Check sheet for the modelled part. Datum: model origin and axes. Units: mm. A direction names the side the tool comes from. Round coordinates to 2 decimals unless told otherwise and drop trailing zeros. Write each loop counter-clockwise with the first axis right and the second up, starting at its lowest first coordinate (ties: lowest second). Pieces come first, ordered by that corner, then holes. Notation, with made-up numbers: (37, 32) -> (73, 32) arc R23 ccw to (73, 64) -> close; hole circle Ø1 at (-28, 80.25). An arc over 180 degrees is marked (long way). One line per item, written item: value.
from build123d import *

# Parameters (mm, degrees)
BOSS_EXTRUDE1_DEPTH = 3.81
BOSS_EXTRUDE3_DEPTH = 21.59
BOSS_EXTRUDE4_DEPTH = 2.54
FILLET1_R           = 2.54
BOSS_EXTRUDE6_DEPTH = 2.54
SKETCH9_R           = 1.905
CUT_EXTRUDE1_DEPTH  = 2.54
CUT_EXTRUDE2_DEPTH  = 1.27
SKETCH11_W          = 22.86
SKETCH11_H          = 2.54
CUT_EXTRUDE3_DEPTH  = 1.27
SKETCH12_W          = 22.86
SKETCH12_H          = 2.54
CUT_EXTRUDE4_DEPTH  = 1.27


with BuildPart() as part:
    # Sketch1 → Boss-Extrude1 (new body)
    with BuildSketch(Plane.XY):
        with BuildLine():
            Line((0, 62.289610149), (0, 73.614735329))
            Line((0, 73.614735329), (-19.541270744, 73.614735329))
            ThreePointArc((-19.541270744, 73.614735329), (-21.690891162, 73.166710129), (-22.687990425, 71.210339105))
            Line((-22.687990425, 71.210339105), (-20.412160003, 5.212586245))
            ThreePointArc((-20.412160003, 5.212586245), (-19.78310781, 3.39559701), (-18.061159176, 2.539998129))
            Line((-18.061159176, 2.539998129), (0, 2.539998129))
            Line((0, 2.539998129), (0, 8.872308918))
            ThreePointArc((0, 8.872308918), (-12.75, 21.622308918), (0, 34.372308918))
            Line((0, 34.372308918), (0, 54.789610149))
            ThreePointArc((0, 54.789610149), (-3.75, 58.539610149), (0, 62.289610149))
        make_face()
        with BuildLine():
            Line((20.141804619, 73.614735329), (0, 73.614735329))
            Line((0, 73.614735329), (0, 62.289610149))
            ThreePointArc((0, 62.289610149), (2.651650429, 61.191260578), (3.75, 58.539610149))
            ThreePointArc((3.75, 58.539610149), (2.651650429, 55.887959719), (0, 54.789610149))
            Line((0, 54.789610149), (0, 34.372308918))
            ThreePointArc((0, 34.372308918), (9.01561146, 30.637920378), (12.75, 21.622308918))
            ThreePointArc((12.75, 21.622308918), (9.01561146, 12.606697458), (0, 8.872308918))
            Line((0, 8.872308918), (0, 2.539998129))
            Line((0, 2.539998129), (17.866078187, 2.539998129))
            ThreePointArc((17.866078187, 2.539998129), (19.630909441, 3.253260423), (20.404569365, 4.992462187))
            Line((20.404569365, 4.992462187), (22.680295797, 70.987199387))
            ThreePointArc((22.680295797, 70.987199387), (21.968542325, 72.839566583), (20.141804619, 73.614735329))
        make_face()
        with BuildLine():
            Line((0, 76.154735329), (-22.77090231, 76.154735329))
            ThreePointArc((-22.77090231, 76.154735329), (-24.597640016, 75.379566583), (-25.309393487, 73.527199387))
            Line((-25.309393487, 73.527199387), (-22.858491178, 2.452464058))
            ThreePointArc((-22.858491178, 2.452464058), (-22.084831254, 0.713262294), (-20.32, 0))
            Line((-20.32, 0), (0, 0))
            Line((0, 0), (0, 2.539998129))
            Line((0, 2.539998129), (-18.061159176, 2.539998129))
            ThreePointArc((-18.061159176, 2.539998129), (-19.78310781, 3.39559701), (-20.412160003, 5.212586245))
            Line((-20.412160003, 5.212586245), (-22.687990425, 71.210339105))
            ThreePointArc((-22.687990425, 71.210339105), (-21.690891162, 73.166710129), (-19.541270744, 73.614735329))
            Line((-19.541270744, 73.614735329), (0, 73.614735329))
            Line((0, 73.614735329), (0, 76.154735329))
        make_face()
        with BuildLine():
            Line((22.77090231, 76.154735329), (0, 76.154735329))
            Line((0, 76.154735329), (0, 73.614735329))
            Line((0, 73.614735329), (20.141804619, 73.614735329))
            ThreePointArc((20.141804619, 73.614735329), (21.968542325, 72.839566583), (22.680295797, 70.987199387))
            Line((22.680295797, 70.987199387), (20.404569365, 4.992462187))
            ThreePointArc((20.404569365, 4.992462187), (19.630909441, 3.253260423), (17.866078187, 2.539998129))
            Line((17.866078187, 2.539998129), (0, 2.539998129))
            Line((0, 2.539998129), (0, 0))
            Line((0, 0), (20.32, 0))
            ThreePointArc((20.32, 0), (22.084831254, 0.713262294), (22.858491178, 2.452464058))
            Line((22.858491178, 2.452464058), (25.309393487, 73.527199387))
            ThreePointArc((25.309393487, 73.527199387), (24.597640016, 75.379566583), (22.77090231, 76.154735329))
        make_face()
    extrude(amount=BOSS_EXTRUDE1_DEPTH)

    # Sketch4 → Boss-Extrude3 (add)
    with BuildSketch(Plane.XY.offset(3.81)):
        with BuildLine():
            Line((-22.77090231, 76.154735329), (22.77090231, 76.154735329))
            ThreePointArc((22.77090231, 76.154735329), (24.597640016, 75.379566583), (25.309393487, 73.527199387))
            Line((25.309393487, 73.527199387), (22.858491178, 2.452464058))
            ThreePointArc((22.858491178, 2.452464058), (22.084831254, 0.713262294), (20.32, 0))
            Line((20.32, 0), (-20.32, 0))
            ThreePointArc((-20.32, 0), (-22.084831254, 0.713262294), (-22.858491178, 2.452464058))
            Line((-22.858491178, 2.452464058), (-25.309393487, 73.527199387))
            ThreePointArc((-25.309393487, 73.527199387), (-24.597640016, 75.379566583), (-22.77090231, 76.154735329))
        make_face()
        with BuildLine():
            Line((-19.541270744, 73.614735329), (20.141804619, 73.614735329))
            ThreePointArc((20.141804619, 73.614735329), (21.968542325, 72.839566583), (22.680295797, 70.987199387))
            Line((22.680295797, 70.987199387), (20.404569365, 4.992462187))
            ThreePointArc((20.404569365, 4.992462187), (19.630909441, 3.253260423), (17.866078187, 2.539998129))
            Line((17.866078187, 2.539998129), (-18.061159176, 2.539998129))
            ThreePointArc((-18.061159176, 2.539998129), (-19.78310781, 3.39559701), (-20.412160003, 5.212586245))
            Line((-20.412160003, 5.212586245), (-22.687990425, 71.210339105))
            ThreePointArc((-22.687990425, 71.210339105), (-21.690891162, 73.166710129), (-19.541270744, 73.614735329))
        make_face(mode=Mode.SUBTRACT)
    extrude(amount=BOSS_EXTRUDE3_DEPTH)

    # Sketch7 → Boss-Extrude4 (add)
    with BuildSketch(Plane.XY.offset(14.605)):
        with BuildLine():
            Line((-19.537731311, 73.614735329), (20.145344052, 73.614735329))
            ThreePointArc((20.145344052, 73.614735329), (21.972081758, 72.839566583), (22.68383523, 70.987199387))
            Line((22.68383523, 70.987199387), (20.408108798, 4.992462187))
            ThreePointArc((20.408108798, 4.992462187), (19.634448874, 3.253260423), (17.86961762, 2.539998129))
            Line((17.86961762, 2.539998129), (-18.057619743, 2.539998129))
            ThreePointArc((-18.057619743, 2.539998129), (-19.730779532, 3.364707915), (-20.389382819, 5.109944754))
            Line((-20.389382819, 5.109944754), (-22.665213241, 71.107697614))
            ThreePointArc((-22.665213241, 71.107697614), (-21.714144758, 73.125513756), (-19.537731311, 73.614735329))
        make_face()
    extrude(amount=BOSS_EXTRUDE4_DEPTH)

    # Fillet1
    fillet1_edges = [part.edges().sort_by_distance(p)[0] for p in [
        (-22.084831254, 0.713262294, 0),
        (-24.083942332, 37.989831723, 0),
        (-24.597640016, 75.379566583, 0),
        (0, 76.154735329, 0),
        (24.597640016, 75.379566583, 0),
        (24.083942332, 37.989831723, 0),
        (22.084831254, 0.713262294, 0),
        (0, 0, 0),
    ]]
    fillet(fillet1_edges, radius=FILLET1_R)

    # Sketch8 → Boss-Extrude6 (add)
    with BuildSketch(Plane.XY.offset(25.4)):
        Polygon((-21.717608556, 43.069831723), (-8.531459132, 43.069831723), (-8.531459132, 32.909831723), (-21.367256671, 32.909831723), align=None)
        Polygon((8.531459132, 32.909831723), (21.367256671, 32.909831723), (21.717608556, 43.069831723), (8.531459132, 43.069831723), align=None)
    extrude(amount=-BOSS_EXTRUDE6_DEPTH)

    # Sketch9 → Cut-Extrude1 (cut)
    with BuildSketch(Plane.XY.offset(25.4)):
        with Locations((-15.036945873, 37.989831723)):
            Circle(SKETCH9_R)
        with Locations(Location((15.237744036, 37.820383377, 0), (0, 0, 180))):
            Circle(SKETCH9_R)
    extrude(amount=-CUT_EXTRUDE1_DEPTH, mode=Mode.SUBTRACT)

    # Sketch10 → Cut-Extrude2 (cut)
    with BuildSketch(Plane(origin=(0, 0, 0), x_dir=(-1, 0, 0), z_dir=(0, 0, -1))):
        Polygon((-21.897084176, 48.274519863), (21.897084176, 48.274519863), (21.809496204, 45.734519863), (-21.809496204, 45.734519863), align=None)
    extrude(amount=-CUT_EXTRUDE2_DEPTH, mode=Mode.SUBTRACT)

    # Sketch11 → Cut-Extrude3 (cut)
    with BuildSketch(Plane(origin=(-22.746873247, -0.784390739, 0), x_dir=(0, 0, 1), z_dir=(-0.9994059754448638, -0.03446296918579016, 0))):
        with Locations((13.97, 47.745550873)):
            Rectangle(SKETCH11_W, SKETCH11_H)
    extrude(amount=-CUT_EXTRUDE3_DEPTH, mode=Mode.SUBTRACT)

    # Sketch12 → Cut-Extrude4 (cut)
    with BuildSketch(Plane(origin=(22.746873247, -0.784390739, 0), x_dir=(0, 0, -1), z_dir=(0.9994059754448638, -0.034462969185789866, 0))):
        with Locations((-13.97, 47.745550873)):
            Rectangle(SKETCH12_W, SKETCH12_H)
    extrude(amount=-CUT_EXTRUDE4_DEPTH, mode=Mode.SUBTRACT)


solid = part.part
Item 1: Release check for a two-part mould opening along Y. For faces 4 (the flat face through (0, 76.155, 14)), 5 (the flat face through (9, 38, 25.4)), 6 (the flat face through (0, 39, 3.81)) record: pulls with the +Y half, pulls with the -Y half, needs draft (parallel to the pull), parting line crosses it, or undercut.
Result set:
face 4: pulls with the +Y half
face 5: needs draft
face 6: undercut
Item 2: Sectioned sample at A-A (z = 12.5). Enter the section's corners in (x, y).
Result set:
outline: (-25.31, 73.53) -> (-24.44, 48.2) -> (-23.17, 48.25) -> (-23.08, 45.71) -> (-24.35, 45.66) -> (-22.86, 2.45) arc R2.54 ccw to (-20.32, 0) -> (20.32, 0) arc R2.54 ccw to (22.86, 2.45) -> (24.35, 45.66) -> (23.08, 45.71) -> (23.17, 48.25) -> (24.44, 48.2) -> (25.31, 73.53) arc R2.54 ccw to (22.77, 76.15) -> (-22.77, 76.15) arc R2.54 ccw to start; hole (-22.69, 71.21) -> (-20.41, 5.21) arc R2.54 ccw to (-18.06, 2.54) -> (17.87, 2.54) arc R2.54 ccw to (20.4, 4.99) -> (22.68, 70.99) arc R2.54 ccw to (20.14, 73.61) -> (-19.54, 73.61) arc R2.54 ccw to start
Item 3: Material ranges on line 1 along Z through (x, y) = (12.5, 36) (3 decimals); line 2 along Y through (x, z) = (-2, 10.75); line 3 along Z through (x, y) = (16, 16) (3 decimals), recorded low to high.
Result set:
line 1: 0 to 3.81, 14.605 to 17.145, 22.86 to 25.4
line 2: 0 to 2.54, 73.61 to 76.15
line 3: 0 to 3.81, 14.605 to 17.145
Item 4: Sectioned sample at B-B (x = 5). Enter the section's corners in (y, z) (3 decimals).
Result set:
outline: (0, 2.54) arc R2.54 ccw to (2.54, 0) -> (9.894, 0) -> (9.894, 3.81) -> (2.54, 3.81) -> (2.54, 14.605) -> (73.615, 14.605) -> (73.615, 3.81) -> (33.351, 3.81) -> (33.351, 0) -> (45.735, 0) -> (45.735, 1.27) -> (48.275, 1.27) -> (48.275, 0) -> (73.615, 0) arc R2.54 ccw to (76.155, 2.54) -> (76.155, 25.4) -> (73.615, 25.4) -> (73.615, 17.145) -> (2.54, 17.145) -> (2.54, 25.4) -> (0, 25.4) -> close
Item 5: Tool access check on faces 1 (the cylindrical face through (19.65, 3.27, 21.21)), 2 (the cylindrical face through (-19.76, 3.37, 14.45)), 3 (the flat face through (0, 0, 14)). Record the directions out of +Z, -Z, +X, -X, +Y, -Y that give a thin tool (end or side, any length) a straight path to the whole face; none if there is none.
Result set:
face 1: +Z
face 2: none
face 3: +Z, -Z, +X, -X, -Y
Item 6: Depth check by flat-ended pin: pin 1 (1.3 mm diameter, centred on y = 36.5, z = 24.5, fed in from +X) (3 decimals); pin 2 (8 mm diameter, centred on y = 8, z = 14, fed in from +X); pin 3 (1 mm diameter, centred on x = -6.5, z = 0.5, fed in from +Y). Enter the tip coordinate at first touch or a pass-through.
Result set:
pin 1: x = 24.055
pin 2: x = 23.19
pin 3: y = 75.63
